For this review, take the finished solid that the model builds, in its own axes (mm). Face numbers are marked on the shaded views. A direction names the side the tool comes from. Give positions to 0.01 mm unless a question says otherwise; leave off trailing zeros. Write each loop counter-clockwise with the first axis right and the second up, starting at its lowest first coordinate (ties: lowest second). Pieces come first, ordered by that corner, then holes. Notation, with made-up numbers: (48.5, -21.5) -> (55.5, -21.5) arc R10 ccw to (55.5, -16.5) -> close; hole circle Ø9 at (49, -39.5). An arc over 180 degrees is marked (long way). Answer as CSV lines item,"result".
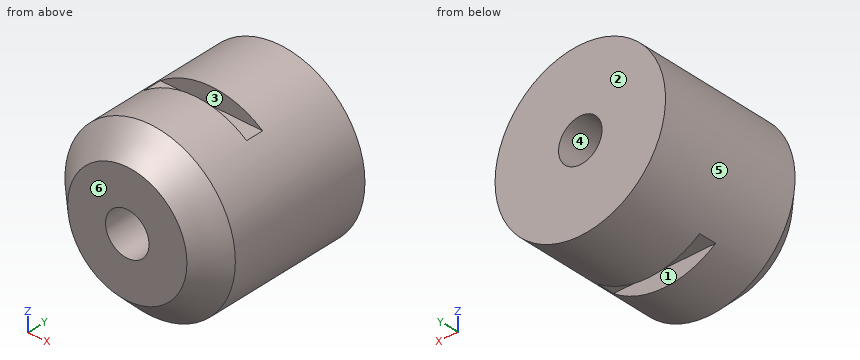
```python
from build123d import *

# Parameters (mm, degrees)
F0_R     = 10
F1_DEPTH = 20
F3_D     = 5.1054
F4_W     = 2.1
F4_H     = 19.5127989389
F5_DEPTH = 12.5
F6_SIZE  = 3


with BuildPart() as f1:
    # F0 (on Front) → F1 (new body)
    with BuildSketch(Plane.XZ):
        Circle(F0_R)
    extrude(amount=F1_DEPTH)

    # F3 (through all)
    with Locations(Plane.XZ.offset(20)):
        with Locations((0, 0)):
            Hole(F3_D / 2)

    # F4 (on Right) → F5 (cut, symmetric)
    with BuildSketch(Plane.YZ):
        with Locations((-10, 17.7563994695)):
            Rectangle(F4_W, F4_H)
        with Locations((-10, -17.7563994695)):
            Rectangle(F4_W, F4_H)
    extrude(amount=F5_DEPTH, both=True, mode=Mode.SUBTRACT)

    # F6
    f6_edges = [f1.edges().sort_by_distance(p)[0] for p in [
        (-10, -20, 0),
    ]]
    chamfer(f6_edges, length=F6_SIZE)


solid = f1.part
```
Q1. Add section B-B (z = 0). Write out the cut boundary in (x, y).
Answer block:
outline,"(-10, -17) -> (-7, -20) -> (-2.55, -20) -> (-2.55, 0) -> (-10, 0) -> close; (2.55, -20) -> (7, -20) -> (10, -17) -> (10, 0) -> (2.55, 0) -> close"
Q2. To check wall thickness, follow probe 1 along Z at (x, y) = (0, -5); probe 2 along Z at (x, y) = (0, -11); probe 3 along X at (y, z) = (-6, 1.5). State the ranges of each line that lie inside material, in increasing order. Write a range as [from, to].
Answer block:
probe 1,"z = [-10, -2.55], [2.55, 10]"
probe 2,"z = [-8, -2.55], [2.55, 8]"
probe 3,"x = [-9.89, -2.07], [2.07, 9.89]"
Q3. Clearance check with flat-ended pins moving along their axes: pin 1 (1.6 mm diameter, centred on x = -1.5, z = 9, fed in from -Y); pin 2 (1.1 mm diameter, centred on x = -0.5, y = -10, fed in from +Z); pin 3 (5 mm diameter, centred on x = 8, y = -7.5, fed in from +Z). State where each tip first meets the part, or that it passes through.
Answer block:
pin 1,"stops at y = -18.68"
pin 2,"stops at z = 8"
pin 3,"stops at z = 8.35"
Q4. Draft analysis for pull direction Z (two halves, no side actions). For the marked faces 4, 5 and 6, state which applies: released by +Z, released by -Z, zero draft, split by the parting line, or undercut.
Answer block:
face 4,"undercut"
face 5,"split by the parting line"
face 6,"zero draft"
Q5. For the marked faces 1, 2 and 3, list the 3-axis set-ups (+Z, -Z, +X, -X, +Y, -Y) from which the entire face can be reached by the end or side of a thin tool; tool diameter is ignored.
Answer block:
face 1,"-Z, +X, -X"
face 2,"+Z, -Z, +X, -X, +Y"
face 3,"+Z, +X, -X"
Q6. Add section C-C (y = -1.5). Write out the cut boundary in (x, z), plus the area to 3 significant figures.
Answer block:
outline,"circle Ø20 at (0, 0); hole circle Ø5.11 at (0, 0)"
area,"294 mm2"
Q7. Add section A-A (x = 0). Write out the cut boundary in (y, z).
Answer block:
outline,"(-20, -7) -> (-17, -10) -> (-11.05, -10) -> (-11.05, -8) -> (-8.95, -8) -> (-8.95, -10) -> (0, -10) -> (0, -2.55) -> (-20, -2.55) -> close; (-20, 2.55) -> (0, 2.55) -> (0, 10) -> (-8.95, 10) -> (-8.95, 8) -> (-11.05, 8) -> (-11.05, 10) -> (-17, 10) -> (-20, 7) -> close"
